Autodesk Inventor part; units mm, degrees
ref_plane "YZ Plane" through (0, 0, 0) normal (1, 0, 0) x (0, 1, 0)
ref_plane "XZ Plane" through (0, 0, 0) normal (0, 1, 0) x (-1, 0, 0)
ref_plane "XY Plane" through (0, 0, 0) normal (0, 0, 1) x (1, 0, 0)
sketch "Sketch1" plane through (0, 0, 0) normal (0, 0, 1) x (1, 0, 0)
  line L0 (-19.603, -9.85) -> (19.603, -9.85)
  line L1 (19.603, -9.85) -> (19.603, 9.85)
  line L2 (19.603, 9.85) -> (-19.603, 9.85)
  line L3 (-19.603, 9.85) -> (-19.603, -9.85)
  line L4 (-19.603, -9.85) -> (19.603, 9.85) construction
  line L5 (19.603, -9.85) -> (-19.603, 9.85) construction
  line L6 (-24.603, 14.85) -> (24.603, 14.85)
  line L7 (24.603, 14.85) -> (24.603, -14.85)
  line L8 (24.603, -14.85) -> (-24.603, -14.85)
  line L9 (-24.603, -14.85) -> (-24.603, 14.85)
  point P0 (0, 0)
  dimension "d0" = 39.206
  dimension "d1" = 19.7
  dimension "d2" = 5
extrude "Extrusion1" add sketch "Sketch1" along normal blind 5
sketch "Sketch2" plane through (0, 0, 5) normal (0, 0, 1) x (1, 0, 0)
  line L0 (-24.603, 14.85) -> (-24.603, -14.85) construction
  line L1 (-24.603, 14.85) -> (-24.603, -14.85) construction
  line L2 (24.603, 14.85) -> (-24.603, 14.85) construction
  line L3 (-24.603, 14.85) -> (24.603, 14.85) construction
  line L4 (24.603, -14.85) -> (24.603, 14.85) construction
  line L5 (24.603, 14.85) -> (24.603, -14.85) construction
  line L6 (24.603, -14.85) -> (-24.603, -14.85) construction
  line L7 (-19.603, -9.85) -> (-19.603, 9.85)
  line L8 (-19.603, 9.85) -> (-24.603, 9.85)
  line L9 (-24.603, 9.85) -> (-24.603, -9.85)
  line L10 (-24.603, -9.85) -> (-19.603, -9.85)
  line L11 (-19.603, -9.85) -> (-19.603, 9.85)
  line L12 (19.603, 9.85) -> (19.603, -9.85)
  line L13 (19.603, 9.85) -> (24.603, 9.85)
  line L14 (24.603, 9.85) -> (24.603, -9.85)
  line L15 (24.603, -9.85) -> (19.603, -9.85)
  line L16 (19.603, -9.85) -> (19.603, 9.85)
  point P0 (0, 0)
extrude "Extrusion2" add sketch "Sketch2" along normal blind 25
sketch "Sketch3" plane through (0, 0, 0) normal (1, 0, 0) x (0, 1, 0)
  circle A0 centre (4.925, 23.111) radius 2.1
  line L0 (14.85, 0) -> (14.85, 5)
  line L1 (14.85, 5) -> (9.85, 5)
  circle A1 centre (-4.925, 23.111) radius 2.1
  line L2 (-14.85, 0) -> (-14.85, 5)
  line L3 (-9.85, 5) -> (-14.85, 5)
  point P0 (0, 0)
  point P1 (-12.35, 5)
  dimension "d7" = 4.2
  dimension "d8" = 9.925
  dimension "d9" = 18.111
  dimension "d10" = 4.2
  dimension "d11" = 9.925
  dimension "d12" = 18.111
extrude "Extrusion3" cut sketch "Sketch3" along normal through all both and the other way through all
sketch "Sketch4" plane through (0, 0, 0) normal (1, 0, 0) x (0, 1, 0)
  line L0 (-9.85, 30) -> (9.85, 30) construction
  line L1 (0, 30) -> (0, 0) construction
  line L2 (24.603, 30) -> (19.603, 30)
  line L3 (19.603, 30) -> (19.603, 25)
  line L4 (19.603, 25) -> (24.603, 25)
  line L5 (24.603, 25) -> (24.603, 30)
  line L6 (14.85, 0) -> (-14.85, 0)
  point P0 (19.603, 27.5)
  dimension "d29" = 5
  dimension "d30" = 5
  dimension "d31" = 19.603
  dimension "d32" = 25
extrude "Extrusion4" add sketch "Sketch4" along normal mid plane 49.206
sketch "Sketch5" plane through (0, 0, 30) normal (0, 0, 1) x (1, 0, 0)
  line L0 (-24.603, -9.85) -> (-24.603, 14.85)
  line L1 (24.603, -9.85) -> (24.603, 14.85)
  line L2 (-24.603, 24.603) -> (24.603, 24.603)
  line L3 (-9.85, 24.603) -> (9.85, 24.603)
  line L4 (9.85, 24.603) -> (9.85, 19.603)
  line L5 (9.85, 19.603) -> (-9.85, 19.603)
  line L6 (-9.85, 19.603) -> (-9.85, 24.603)
  line L7 (24.603, 24.603) -> (24.603, 19.603)
  line L8 (-24.603, 19.603) -> (-24.603, 24.603)
  point P0 (0, 0)
  point P1 (9.85, 22.103)
  point P2 (-24.603, 22.103)
  point P3 (9.85, 24.603)
  dimension "d33" = 19.7
  dimension "d34" = 5
  dimension "d35" = 14.753
  dimension "d36" = 14.753
extrude "Extrusion5" add sketch "Sketch5" along normal blind 30
sketch "Sketch7" plane through (19.603, 9.85, 5) normal (0, 1, 0) x (1, 0, 0)
  line L0 (-39.206, 0) -> (-39.206, -25)
  line L1 (-39.206, -25) -> (-44.206, -25)
  line L2 (-44.206, -25) -> (-44.206, -20)
  line L3 (-44.206, -20) -> (-39.206, -20)
  line L4 (-39.206, -20) -> (-39.206, -25)
  line L5 (0, 0) -> (0, -25)
  line L6 (0, -25) -> (5, -25)
  line L7 (5, -25) -> (5, -20)
  line L8 (5, -20) -> (0, -20)
  line L9 (0, -20) -> (0, -25)
  point P0 (-19.603, 5)
  dimension "d37" = 5
  dimension "d38" = 5
  dimension "d39" = 5
  dimension "d40" = 5
extrude "Extrusion7" add sketch "Sketch7" along normal through all
sketch "Sketch8" plane through (-24.603, 24.603, 25) normal (0, 1, 0) x (1, 0, 0)
  line L0 (14.753, -35) -> (34.453, -35) construction
  line L1 (24.603, -35) -> (24.603, 0) construction
  line L2 (5, 0) -> (44.206, 0) construction
  circle A0 centre (24.603, -27) radius 3
  point P0 (24.603, 25)
  dimension "d43" = 6
  dimension "d44" = 8
extrude "Extrusion8" cut sketch "Sketch8" against normal through all
fillet "Fillet1" radius 9.85 2 edges at (9.85, 22.103, 60) (-9.85, 22.103, 60)
properties part number "Part2_cage"
Geometry: final body of the model. Coordinates: model frame, mm. A direction names the side the tool comes from. Coordinates: 2 decimals unless noted, no trailing zeros. Loops run counter-clockwise (first coordinate to the right, second up) from the corner with the lowest first, then second, coordinate; pieces in that order, holes last. Notation, with made-up numbers: M 61.5,53 L 106.5,53 A32 cw 106.5,81 Z; hole C 27.5,61 d10. An arc over 180 degrees is marked long. One line per item, written item: value. Start each with the question number.
1) Reachability of faces 1 (the flat face through (22, -9.85, 17)), 2 (the cylindrical face through (22.07, -5.38, 25.16)), 3 (the flat face through (-9.85, 22, 40)), 4 (the flat face through (9.85, 22, 40)), 5 (the flat face through (0, -9.85, 2)) from +Z, -Z, +X, -X, +Y, -Y: full face, straight path, thin tool, end or side. Return the list, or none.
2) Cut plane C-C (y = -1). Return loops of the section in (x, z).
3) Cut plane B-B (x = 16). Return loops of the section in (y, z), then the cut area to 3 significant figures.
4) Cut plane A-A (y = 11). Return loops of the section in (x, z), then the cut area to 3 significant figures.
5) Material intervals for L1, parallel to X at y = 0.5, z = 20; L2, parallel to Y at x = 8.5, z = 4; L3, parallel to Z at x = -15, y = 22.5, sorted ascending. Write a range as from..to.
6) Draft query along X for faces 6 (the flat face through (0, 19.603, 39)), 7 (the flat face through (24.603, 0, 15)), 8 (the flat face through (0, 14.85, 2)). Return one class per face: released by +X, released by -X, zero draft, split by the parting line, or undercut.
7) Pin query (flat end, axial travel): P1, Ø3, axis at x = 4, z = 22, coming from the +Y side; P2, Ø4, axis at x = -22, z = 14, coming from the +Y side; P3, Ø1.5, axis at x = 12, z = 3.5, coming from the +Y side; P4, Ø4, axis at x = -2, y = 11.5, coming from the -Z side. Return the tip coordinate at first contact, or that it passes through.
Evaluation:
1. face 1: +Z, +X, -X, -Y
1. face 2: +X, -X
1. face 3: +Z, -X, +Y, -Y
1. face 4: +Z, +X, +Y, -Y
1. face 5: +Z, -Z
2. outline: M -24.6,0 L -19.6,0 L -19.6,30 L -24.6,30 Z; M 19.6,0 L 24.6,0 L 24.6,30 L 19.6,30 Z
3. outline: M -14.85,0 L -9.85,0 L -9.85,5 L -14.85,5 Z; M 9.85,0 L 14.85,0 L 14.85,5 L 9.85,5 Z; M 19.6,25 L 24.6,25 L 24.6,30 L 19.6,30 Z
3. area: 75.0 mm^2
4. outline: M -24.6,0 L 24.6,0 L 24.6,5 L -24.6,5 Z; M -24.6,25 L -19.6,25 L -19.6,30 L -24.6,30 Z; M 19.6,25 L 24.6,25 L 24.6,30 L 19.6,30 Z
4. area: 296 mm^2
5. L1: -24.6..-19.6, 19.6..24.6
5. L2: -14.85..-9.85, 9.85..14.85
5. L3: 25..30
6. face 6: undercut
6. face 7: released by +X
6. face 8: zero draft
7. P1: through
7. P2: y = 9.85
7. P3: y = 14.85
7. P4: z = 0
